```python
from build123d import *

# Parameters (mm, degrees)
SKETCH1_W           = 80
SKETCH1_H           = 70
BOSS_EXTRUDE1_DEPTH = 50
SKETCH2_W           = 20
SKETCH2_H           = 20
CUT_EXTRUDE1_DEPTH  = 51


with BuildPart() as part:
    # Sketch1 → Boss-Extrude1 (new body)
    with BuildSketch(Plane(origin=(0, 0, 0), x_dir=(1, 0, 0), z_dir=(0, 1, 0))):
        Rectangle(SKETCH1_W, SKETCH1_H)
        Polygon((40, 35), (40, 85), (-40, 35), align=None)
    extrude(amount=BOSS_EXTRUDE1_DEPTH)

    # Sketch2 → Cut-Extrude1 (cut, through all)
    with BuildSketch(Plane(origin=(0, 50, 0), x_dir=(1, 0, 0), z_dir=(0, 1, 0))):
        Rectangle(SKETCH2_W, SKETCH2_H)
    extrude(amount=-CUT_EXTRUDE1_DEPTH, mode=Mode.SUBTRACT)


solid = part.part
```
Source: CAD feature listing. Evaluate the final solid. Frame: model axes, mm. A direction names the side the tool comes from. Coordinates: 2 decimals unless noted, no trailing zeros. Loops run counter-clockwise (first coordinate to the right, second up) from the corner with the lowest first, then second, coordinate; pieces in that order, holes last. Notation, with made-up numbers: M 72.5,-5 L 79.5,-5 A22 ccw 79.5,32 Z; hole C 84.5,-30 d9. An arc over 180 degrees is marked long. Use a Markdown table: item, result. Add a question column.
Q1. Material intervals for L1, parallel to X at y = 18.5, z = -1.5; L2, parallel to Z at x = -9, y = 41.5 (3 decimals); L3, parallel to Z at x = -9.5, y = 40.5, sorted ascending.
Q2. First-contact query: pin 1 (10 mm diameter, centred on x = -5, z = -15.5, fed in from -Y); pin 2 (8 mm diameter, centred on y = 5, z = -47.5, fed in from -X); pin 3 (8 mm diameter, centred on x = -21, y = 38.5, fed in from -Z) (3 decimals); pin 4 (1 mm diameter, centred on x = -23.5, y = 31, fed in from -Z) (3 decimals). Flat tips, straight axial feed; report the tip coordinate or a pass-through.
Q3. Draft query along X for faces 3 (the flat face through (40, 25, -24)), 4 (the flat face through (0.56, 24.65, -60.35)), 5 (the flat face through (0, 25, 10)), 6 (the flat face through (-1, 0, -13)). Return one class per face: pulls with the +X half, pulls with the -X half, needs draft (parallel to the pull), parting line crosses it, or undercut.
Q4. Section query D-D, the plane x = 18. Return loops of the section in (y, z).
Q5. Section query A-A, the plane z = -5. Return loops of the section in (x, y).
Q6. Access query for faces 1 (the flat face through (-10, 25, 0)), 2 (the flat face through (-1, 25, 35)). Directions: +Z, -Z, +X, -X, +Y, -Y. A direction counts if a zero-diameter tool reaches every point of the face in a straight line with its end or side. Return the directions, or none.
Q7. Section query C-C, the plane x = -7.5. Return loops of the section in (y, z), and give its area (3 significant figures).
Q8. Section query B-B, the plane y = 7. Return loops of the section in (x, z), and give its area (3 significant figures).
Result:
| question | item | result |
|---|---|---|
| 1 | L1 | x = -40 to -10, 10 to 40 |
| 1 | L2 | z = -54.375 to -10, 10 to 35 |
| 1 | L3 | z = -54.06 to -10, 10 to 35 |
| 2 | pin 1 | stops at y = 0 |
| 2 | pin 2 | stops at x = -26.4 |
| 2 | pin 3 | stops at z = -49.375 |
| 2 | pin 4 | stops at z = -45.625 |
| 3 | face 3 | pulls with the +X half |
| 3 | face 4 | pulls with the -X half |
| 3 | face 5 | undercut |
| 3 | face 6 | needs draft |
| 4 | outline | M 0,-71.25 L 50,-71.25 L 50,35 L 0,35 Z |
| 5 | outline | M -40,0 L -10,0 L -10,50 L -40,50 Z; M 10,0 L 40,0 L 40,50 L 10,50 Z |
| 6 | face 1 | +Y, -Y |
| 6 | face 2 | +Z, +X, -X, +Y, -Y |
| 7 | outline | M 0,-55.31 L 50,-55.31 L 50,-10 L 0,-10 Z; M 0,10 L 50,10 L 50,35 L 0,35 Z |
| 7 | area | 3,520 mm2 |
| 8 | outline | M -40,-35 L 40,-85 L 40,35 L -40,35 Z; hole M -10,-10 L 10,-10 L 10,10 L -10,10 Z |
| 8 | area | 7,200 mm2 |
